Could you check a few things on this model? Use its own coordinates, in mm. Give positions to 0.01 mm unless a question says otherwise; leave off trailing zeros. Loops run counter-clockwise (first coordinate to the right, second up) from the corner with the lowest first, then second, coordinate; pieces in that order, holes last. Notation, with made-up numbers: M 37.25,-24.5 L 85.25,-24.5 A23 ccw 85.25,11.5 Z; hole C -30.75,40.25 d1. An arc over 180 degrees is marked long. Answer in a Markdown table with one row per item. Add a question column.
1. If we section it at B-B on x = -32: List the corners of the cut face in (y, z) for me, then the cut area to 3 significant figures.
2. If we section it at C-C on y = 4.5: List the corners of the cut face in (x, z) for me, then the cut area to 3 significant figures.
3. I need wall thicknesses on line 1 along Y through (x, z) = (3, 263); line 2 along Y through (x, z) = (-6, 67); line 3 along X through (y, z) = (6.75, 304). Which ranges of each line are inside material? Lowest first, please. Write a range as from..to.
4. If we section it at A-A on z = 508: List the corners of the cut face in (x, y) for me, then the cut area to 3 significant figures.
5. I'm going to push flat-ended pins straight in: pin 1 Ø4 at (x, z) = (23.5, 224) entering from +Y; pin 2 Ø2 at (y, z) = (-1.5, 207) entering from +X; pin 3 Ø5 at (x, z) = (-28.5, 92.5) entering from +Y. Where does each tip first touch, or does it pass through?
```python
from build123d import *

# Parameters (mm, degrees)
F0_W      = 79.5655027032
F0_H      = 36.2267494202
F1_DEPTH  = 12.7
F2_DEPTH  = 12.7
F4_DEPTH  = 508
F7_DEPTH  = 76.2
F8_SIZE2  = 59.4614
F8_SIZE   = 15.9326341108
F9_DEPTH  = 25.4
F10_DEPTH = 25.4
F12_DEPTH = 990.6


with BuildPart() as f1:
    # F0 (on Top) → F1 (new body)
    with BuildSketch(Plane.XY):
        with Locations((-0.5556233227, -0.4444997758)):
            Rectangle(F0_W, F0_H)
    extrude(amount=F1_DEPTH)

    # F2 (add): a face of the model
    f2_faces = [f1.faces().sort_by_distance(p)[0] for p in [
        (-0.5556233227, -0.4444997758, 0),
    ]]
    extrude(f2_faces, amount=F2_DEPTH)

    # F3 (on face) → F4 (join)
    with BuildSketch(Plane.XY.offset(12.7)):
        Polygon((-39.5987667143, 0), (0, -17.9184600711), (38.5859385133, 0), (0, 16.9973578304), align=None)
    extrude(amount=F4_DEPTH)

    # F5 (on face) → F7 (join)
    with BuildSketch(Plane.XY.offset(520.7)):
        Polygon((0, 16.9973578304), (-39.5987667143, 0), (0, -17.9184600711), (38.5859385133, 0), align=None)
    extrude(amount=F7_DEPTH)

    # F8
    f8_edges = [f1.edges().sort_by_distance(p)[0] for p in [
        (-19.799383, 8.498679, 596.9),
        (-19.799383, -8.95923, 596.9),
        (19.292969, -8.95923, 596.9),
        (19.292969, 8.498679, 596.9),
    ]]
    f8_side = f1.faces().sort_by_distance((-0.337609, -0.307034, 596.9))[0]
    chamfer(f8_edges, length=F8_SIZE, length2=F8_SIZE2, reference=f8_side)

    # F9 (cut): a face of the model
    f9_faces = [f1.faces().sort_by_distance(p)[0] for p in [
        (-0.5556233227, 17.6688749343, 0),
    ]]
    extrude(f9_faces, amount=-F9_DEPTH, mode=Mode.SUBTRACT)

    # F10 (cut): a face of the model
    f10_faces = [f1.faces().sort_by_distance(p)[0] for p in [
        (-0.5556233227, -18.5578744859, 0),
    ]]
    extrude(f10_faces, amount=-F10_DEPTH, mode=Mode.SUBTRACT)

    # F11 (on face) → F12 (cut)
    with BuildSketch(Plane(origin=(0, 0, 12.7), x_dir=(1, 0, 0), z_dir=(0, 0, -1))):
        Polygon((19.2929692566, -8.4986789152), (-19.0062443799, -8.8391255534), (0, -16.9973578304), align=None)
        Polygon((0, 17.9184600711), (-19.7993833572, 8.9592300355), (19.2929692566, 8.9592300355), align=None)
    extrude(amount=-F12_DEPTH, mode=Mode.SUBTRACT)


solid = f1.part
```
Results:
| question | item | result |
|---|---|---|
| 1 | outline | M -3.44,12.7 L 3.26,12.7 L 3.26,537.44 L -0.07,548.88 L -3.44,537.44 Z |
| 1 | area | 3,550 mm2 |
| 2 | outline | M -29.12,12.7 L 28.37,12.7 L 28.37,537.44 L -0.06,580.21 L -29.12,537.44 Z |
| 2 | area | 31,400 mm2 |
| 3 | line 1 | -8.96..8.64 |
| 3 | line 2 | -8.96..8.72 |
| 3 | line 3 | -23.87..23.26 |
| 4 | outline | M -39.6,0 L -19.8,-8.96 L 19.29,-8.96 L 38.59,0 L 19.29,8.5 L -19.01,8.84 Z |
| 4 | area | 1,030 mm2 |
| 5 | pin 1 | y = 7.53 |
| 5 | pin 2 | x = 37.51 |
| 5 | pin 3 | y = 5.84 |
